Read the model definition and answer for the solid it produces. Units are mm, in the model's axes. A direction names the side the tool comes from. Give positions to 0.01 mm unless a question says otherwise; leave off trailing zeros. Order: outer loops, then holes, each group sorted by start corner. A loop starts at its lowest first (then second) coordinate and runs counter-clockwise, first axis right, second up.
```python
from build123d import *

# Parameters (mm, degrees)
F1_DEPTH       = 111
F2_W           = 70.5
F2_H           = 10
F3_DEPTH       = 105.2
F5_DEPTH       = 150
F7_D           = 3.3
F7_DEPTH       = 5
F7_CBORE_D     = 6.5
F7_CBORE_DEPTH = 0.5
F7_TIP         = 0.9914200214
F9_D           = 3.3
F9_DEPTH       = 5
F9_CBORE_D     = 6.5
F9_CBORE_DEPTH = 0.5
F9_TIP         = 0.9914200214
F11_START      = 25
F11_DEPTH      = 25
F12_R          = 1
F14_DEPTH      = 5


with BuildPart() as f1:
    # F0 (on Front) → F1 (new body)
    with BuildSketch(Plane.XZ):
        Polygon((73, 19), (0, 19), (0, 5), (9, 0), (64, 0), (73, 5), align=None)
    extrude(amount=F1_DEPTH)

    # F2 (on Front) → F3 (cut)
    with BuildSketch(Plane.XZ):
        with Locations((36.5, 11)):
            Rectangle(F2_W, F2_H)
    extrude(amount=F3_DEPTH, mode=Mode.SUBTRACT)

    # F4 (on Front) → F5 (cut)
    with BuildSketch(Plane.XZ):
        with BuildLine():
            Line((41.5, 19), (31.5, 19))
            Line((31.5, 19), (31.5, 8))
            ThreePointArc((31.5, 8), (36.5, 6.1897503241), (41.5, 8))
            Line((41.5, 8), (41.5, 19))
        make_face()
    extrude(amount=F5_DEPTH, mode=Mode.SUBTRACT)

    # F7
    with Locations(Plane(origin=(0, 0, 0), x_dir=(0, 1, 0), z_dir=(-1, 0, 0))):
        with Locations((-95, -9.2), (-18.2, -9.2)):
            CounterBoreHole(F7_D / 2, F7_CBORE_D / 2, F7_CBORE_DEPTH, depth=F7_DEPTH)
            with Locations((0, 0, -(F7_DEPTH + F7_TIP / 2))):  # 118° drill point
                Cone(0, F7_D / 2, F7_TIP, mode=Mode.SUBTRACT)

    # F9
    with Locations(Plane.YZ.offset(73)):
        with Locations((-95, 9.2), (-18.2, 9.2)):
            CounterBoreHole(F9_D / 2, F9_CBORE_D / 2, F9_CBORE_DEPTH, depth=F9_DEPTH)
            with Locations((0, 0, -(F9_DEPTH + F9_TIP / 2))):  # 118° drill point
                Cone(0, F9_D / 2, F9_TIP, mode=Mode.SUBTRACT)

    # F10 (on Right) → F11 (cut)
    with BuildSketch(Plane.YZ.offset(F11_START)):
        with BuildLine():
            Line((-99.916331174, 4.5), (-105.1256978151, 4.5))
            ThreePointArc((-105.1256978151, 4.5), (-105.7839048332, 4.2528369819), (-106.1167429851, 3.6335270426))
            Line((-106.1167429851, 3.6335270426), (-106.6063010141, 0))
            Line((-106.6063010141, 0), (-104.1063010141, 0))
            Line((-104.1063010141, 0), (-104.1063010141, 1.5))
            ThreePointArc((-104.1063010141, 1.5), (-103.8134077953, 2.2071067812), (-103.1063010141, 2.5))
            Line((-103.1063010141, 2.5), (-102.1063010141, 2.5))
            ThreePointArc((-102.1063010141, 2.5), (-101.3991942329, 2.2071067812), (-101.1063010141, 1.5))
            Line((-101.1063010141, 1.5), (-101.1063010141, 0))
            Line((-101.1063010141, 0), (-98.6063010141, 0))
            Line((-98.6063010141, 0), (-98.9201364759, 3.5871557427))
            ThreePointArc((-98.9201364759, 3.5871557427), (-99.2407409664, 4.2372773368), (-99.916331174, 4.5))
        make_face()
    extrude(amount=F11_DEPTH, mode=Mode.SUBTRACT)

    # F12
    f12_edges = [f1.edges().sort_by_distance(p)[0] for p in [
        (73, -55.5, 19),
        (0, -55.5, 19),
        (31.5, -55.5, 19),
        (41.5, -55.5, 19),
        (9, -55.5, 0),
        (64, -55.5, 0),
        (73, -55.5, 5),
        (0, -55.5, 5),
    ]]
    fillet(f12_edges, radius=F12_R)

    # F13 (on face) → F14 (cut)
    with BuildSketch(Plane(origin=(0, 0, 0), x_dir=(-1, 0, 0), z_dir=(0, 1, 0))):
        with BuildLine():
            Line((-18.35, 6), (-65.35, 6))
            Line((-65.35, 6), (-65.35, 3.2))
            ThreePointArc((-65.35, 3.2), (-65.0571067812, 2.4928932188), (-64.35, 2.2))
            Line((-64.35, 2.2), (-19.35, 2.2))
            ThreePointArc((-19.35, 2.2), (-18.6428932188, 2.4928932188), (-18.35, 3.2))
            Line((-18.35, 3.2), (-18.35, 6))
        make_face()
    extrude(amount=-F14_DEPTH, mode=Mode.SUBTRACT)


solid = f1.part
```
1) The part is cut by section A-A on z = 9.2. Count the separate pieces of the cut face and the enclosed holes in it, and give its area (4 significant figures).
Final values:
separate pieces: 6
enclosed holes: 0
area: 605.5 mm2
2) The part is cut by section B-B on y = -65.5. Determine the outline of the cut face in (x, z).
Final values:
outline: (0, 5.59) arc R1 ccw to (0.51, 4.71) - (8.77, 0.13) arc R1 ccw to (9.26, 0) - (63.74, 0) arc R1 ccw to (64.23, 0.13) - (72.49, 4.71) arc R1 ccw to (73, 5.59) - (73, 18) arc R1 ccw to (72, 19) - (42.5, 19) arc R1 ccw to (41.5, 18) - (41.5, 16) - (71.75, 16) - (71.75, 6) - (1.25, 6) - (1.25, 16) - (31.5, 16) - (31.5, 18) arc R1 ccw to (30.5, 19) - (1, 19) arc R1 ccw to (0, 18) - close
3) A tool of negligible diameter and unlimited length cuts with its end or side. For faces 1 (the face through (1.25, -52, 11)), 2 (the face through (72.5, -96, 11)), 3 (the face through (37, -102, 4.5)), 4 (the face through (0.246, -98.247, 9.057)), from which of +Z, -Z, +X, -X, +Y, -Y can it reach the whole face along a straight path? Write none if from no direction.
Final values:
face 1: +Y
face 2: +X
face 3: none
face 4: -X
4) For a pull along Z with two mould halves and no side action, classify faces 5 (the face through (73, -55, 12)), 6 (the face through (42, -2, 2.2)), 7 (the face through (36.42, -108.06, 6.19)), 8 (the face through (36, -55, 0)) as released by +Z, released by -Z, zero draft, split by the parting line, or undercut.
Final values:
face 5: zero draft
face 6: undercut
face 7: released by +Z
face 8: released by -Z
5) The part is cut by section C-C on x = 56.5. Determine the outline of the cut face in (y, z), and give its area (3 significant figures).
Final values:
outline: (-111, 0) - (0, 0) - (0, 2.2) - (-5, 2.2) - (-5, 6) - (-105.2, 6) - (-105.2, 16) - (0, 16) - (0, 19) - (-111, 19) - close
area: 1,040 mm2
6) Given pin 1 (7 mm diameter, centred on y = -95, z = 8.5, fed in from +X); pin 2 (2 mm diameter, centred on x = 43, z = 12, fed in from +Y); pin 3 (0.8 mm diameter, centred on x = 36, y = -102.5, fed in from +Z); pin 4 (2 mm diameter, centred on y = -3, z = 4.5, fed in from -X), each flat-ended and moving along its own axis, determine where each tip first touches the part or whether it passes through.
Final values:
pin 1: stops at x = 73
pin 2: stops at y = -105.2
pin 3: stops at z = 6
pin 4: stops at x = 0
7) Consider L1, parallel to Y at x = 0.95, z = 9.2; L2, parallel to Z at x = 20, y = -71.5; L3, parallel to X at y = -22.5, z = 9.5. Determine where each line is inside the solid, lowest interval first.
Final values:
L1: y = -111 to -96.65, -93.35 to -19.85, -16.55 to 0
L2: z = 0 to 6, 16 to 19
L3: x = 0 to 1.25, 71.75 to 73
